Geometry: see drawing. Coordinates: mm, zero at the bounding-box minimum. Round coordinates to 2 decimals unless told otherwise and drop trailing zeros. Loops run counter-clockwise (first coordinate to the right, second up) from the corner with the lowest first, then second, coordinate; pieces in that order, holes last.
(1) Material intervals for probe 1 along X at (y, z) = (4, 17.5) (1 decimal); probe 2 along Z at (x, y) = (35.5, 3.25) (1 decimal); probe 3 along Z at (x, y) = (56, 4) (1 decimal), sorted ascending.
(2) Section A-A, the plane z = 36. Return the cut outline in (x, y).
(3) Section C-C, the plane y = 2.5. Count the separate pieces of the cut face and the enclosed holes in it, plus the area to 3 significant figures.
(4) Mould query, pull axis Z, two halves, no side actions, for the marked faces 1, 2 and 3. Classes: pulls with the +Z half, pulls with the -Z half, needs draft (parallel to the pull), parting line crosses it, or undercut.
(5) First-contact query: pin 1 Ø1 at (y, z) = (5.5, 31) entering from -X (1 decimal); pin 2 Ø3 at (x, y) = (16, 3.5) entering from +Z (1 decimal). Flat tips, straight axial feed; report the tip coordinate or a pass-through.
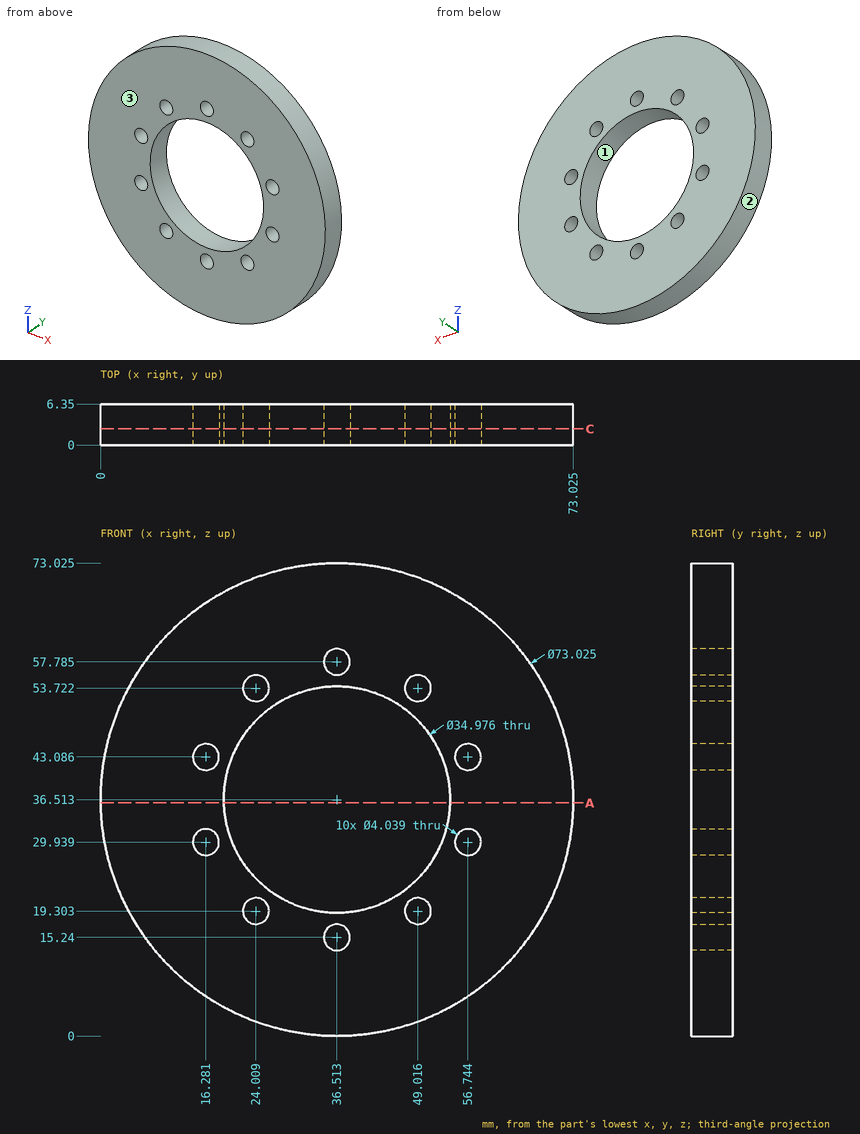
Output values:
1. probe 1: x = 5.3 to 23.1, 24.9 to 48.1, 49.9 to 67.7
1. probe 2: z = 0 to 13.5, 17 to 19.1, 54 to 56, 59.5 to 73
1. probe 3: z = 5.6 to 28.1, 31.8 to 41.2, 45 to 67.4
2. outline: (0, 0) - (19.03, 0) - (19.03, 6.35) - (0, 6.35) - close; (53.99, 0) - (73.02, 0) - (73.02, 6.35) - (53.99, 6.35) - close
3. separate pieces: 1
3. enclosed holes: 11
3. area: 3,100 mm2
4. face 1: undercut
4. face 2: parting line crosses it
4. face 3: needs draft
5. pin 1: stops at x = 0.3
5. pin 2: stops at z = 67.7
